from build123d import *

# Parameters (mm, degrees)
SKETCH1_R           = 9
BOSS_EXTRUDE1_DEPTH = 12.5
CUT_EXTRUDE1_START  = -12.5
SKETCH2_R           = 4
CUT_EXTRUDE1_DEPTH  = 12.5
CUT_EXTRUDE2_REACH  = 30.054
SKETCH3_R           = 2.5


with BuildPart() as part:
    # Sketch1 → Boss-Extrude1 (new, symmetric)
    with BuildSketch(Plane(origin=(0, 0, 0), x_dir=(1, 0, 0), z_dir=(0, 1, 0))):
        with Locations(Location((0, 0, 0), (0, 0, 270))):
            Circle(SKETCH1_R)
    extrude(amount=BOSS_EXTRUDE1_DEPTH, both=True)

    # Sketch2 → Cut-Extrude1 (cut)
    with BuildSketch(Plane(origin=(0, 12.5, 0), x_dir=(1, 0, 0), z_dir=(0, 1, 0)).offset(CUT_EXTRUDE1_START)):
        with Locations(Location((0, 0, 0), (0, 0, 270))):
            Circle(SKETCH2_R)
    extrude(amount=CUT_EXTRUDE1_DEPTH, mode=Mode.SUBTRACT)

    # Sketch3 → Cut-Extrude2 (cut, up to next)
    with BuildSketch(Plane.XZ.offset(12.5), mode=Mode.PRIVATE) as cut_extrude2_sk1:
        with Locations(Location((0, 0, 0), (0, 0, 270))):
            Circle(SKETCH3_R)
    cut_extrude2_tool1 = extrude(cut_extrude2_sk1.sketch, amount=-CUT_EXTRUDE2_REACH, mode=Mode.PRIVATE) & part.part
    add(cut_extrude2_tool1.solids().sort_by_distance((0, -12.5, 0))[0], mode=Mode.SUBTRACT)


solid = part.part
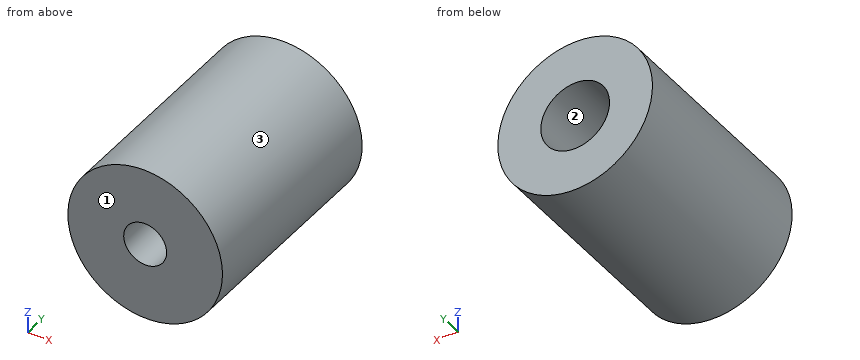
The listing builds one solid part. Answer for the finished solid, in the listing's coordinates (mm). Face numbers are marked on the shaded views. Coordinates: 2 decimals unless noted, no trailing zeros. Order: outer loops, then holes, each group sorted by start corner. A loop starts at its lowest first (then second) coordinate and runs counter-clockwise, first axis right, second up. Notation, with made-up numbers: (35.25, 89.5) -> (87.25, 89.5) arc R7 ccw to (87.25, 96.5) -> close; hole circle Ø3 at (-7.75, 87.25). An arc over 180 degrees is marked (long way). Answer in a Markdown table with one row per item. Add a question column.
Item 1: Determine the mould class of the marked faces 1, 2 and 3 for opening direction Z: +Z half, -Z half, draft (parallel to the pull), parting line (faces both ways), or undercut.
Item 2: Each of these flat-tipped pins is pushed along its axis until it touches: P1, Ø4, axis at y = 0.5, z = 6, coming from the +X side; P2, Ø1, axis at x = -4.5, y = 8, coming from the +Z side; P3, Ø7, axis at x = 0, z = 0, coming from the +Y side. Where does it stop, or does it pass through?
Item 3: Find section B-B (x = 0). Write down the section's boundary in (y, z), then the cut area to 4 significant figures.
Item 4: Find the intervals of material crossed by L1, parallel to X at y = -7, z = 0; L2, parallel to X at y = 6, z = 0; L3, parallel to Y at x = 2.75, z = 1, in increasing order. Write a range as from..to.
Item 5: Find section D-D (z = 3.5). Write down the section's boundary in (x, y), then the cut area to 3 significant figures.
Item 6: Find section C-C (y = 7.5). Write down the section's boundary in (x, z).
Item 7: Find section A-A (z = 0). Write down the section's boundary in (x, y).
Result set:
| question | item | result |
|---|---|---|
| 1 | face 1 | draft |
| 1 | face 2 | undercut |
| 1 | face 3 | parting line |
| 2 | P1 | stops at x = 8.06 |
| 2 | P2 | stops at z = 8.06 |
| 2 | P3 | stops at y = 0 |
| 3 | outline | (-12.5, -9) -> (12.5, -9) -> (12.5, -4) -> (0, -4) -> (0, -2.5) -> (-12.5, -2.5) -> close; (-12.5, 2.5) -> (0, 2.5) -> (0, 4) -> (12.5, 4) -> (12.5, 9) -> (-12.5, 9) -> close |
| 3 | area | 287.5 mm² |
| 4 | L1 | x = -9..-2.5, 2.5..9 |
| 4 | L2 | x = -9..-4, 4..9 |
| 4 | L3 | y = -12.5..0 |
| 5 | outline | (-8.29, -12.5) -> (8.29, -12.5) -> (8.29, 12.5) -> (1.94, 12.5) -> (1.94, 0) -> (-1.94, 0) -> (-1.94, 12.5) -> (-8.29, 12.5) -> close |
| 5 | area | 366 mm² |
| 6 | outline | circle Ø18 at (0, 0); hole circle Ø8 at (0, 0) |
| 7 | outline | (-9, -12.5) -> (-2.5, -12.5) -> (-2.5, 0) -> (-4, 0) -> (-4, 12.5) -> (-9, 12.5) -> close; (2.5, -12.5) -> (9, -12.5) -> (9, 12.5) -> (4, 12.5) -> (4, 0) -> (2.5, 0) -> close |
